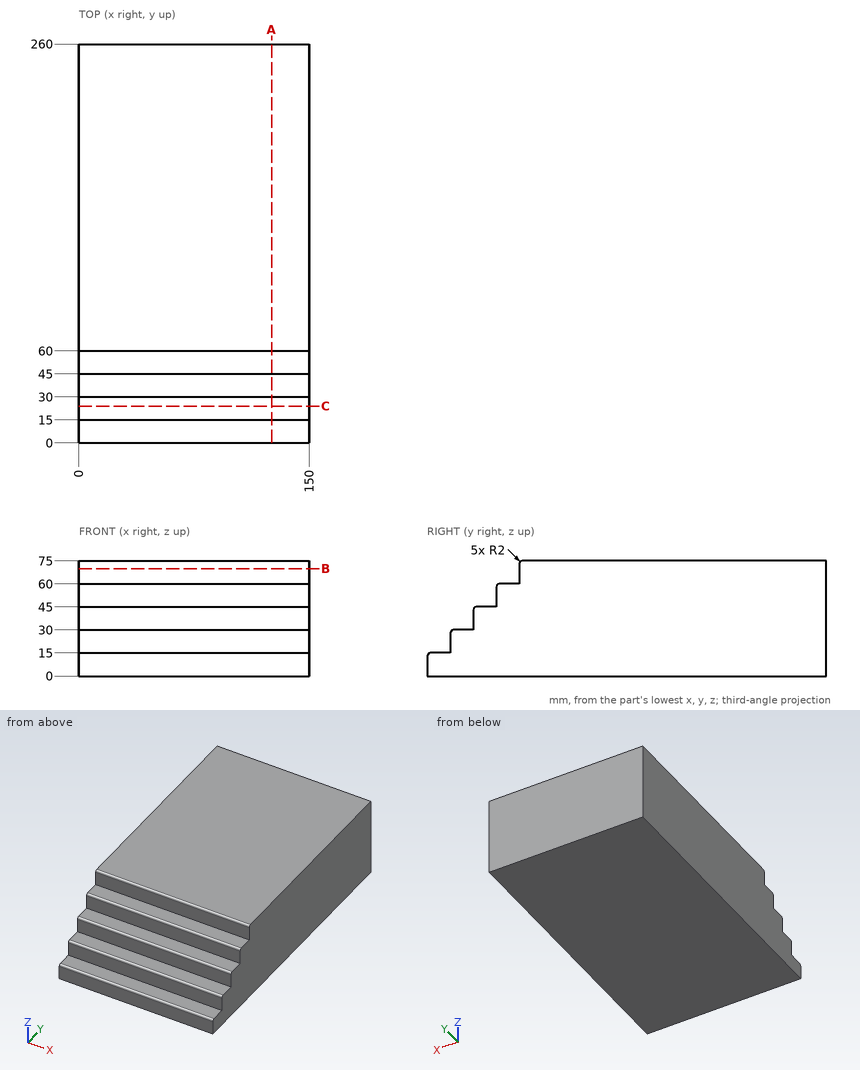
Geometry: see drawing. Coordinates: mm, zero at the bounding-box minimum. Round coordinates to 2 decimals unless told otherwise and drop trailing zeros. Write each loop counter-clockwise with the first axis right and the second up, starting at its lowest first coordinate (ties: lowest second). Pieces come first, ordered by that corner, then holes.
Item 1: Section query B-B (z = 70). Return loops of the section in (x, y), plus the area to 3 significant figures.
Item 2: Material intervals for L1, parallel to Y at x = 113.5, z = 17; L2, parallel to Y at x = 45.5, z = 71.5; L3, parallel to Z at x = 71, y = 32, sorted ascending.
Item 3: Section query A-A (x = 125.5). Return loops of the section in (y, z), plus the area to 3 significant figures.
Item 4: Section query C-C (y = 24). Return loops of the section in (x, z), plus the area to 3 significant figures.
Item 5: Pin query (flat end, axial travel): P1, Ø12, axis at x = 56.5, z = 39.5, coming from the -Y side; P2, Ø10.5, axis at x = 50.5, z = 68.5, coming from the -Y side; P3, Ø14.5, axis at x = 39, y = 11.5, coming from the +Z side. Return the tip coordinate at first contact, or that it passes through.
Completed:
1. outline: (0, 60) - (150, 60) - (150, 260) - (0, 260) - close
1. area: 30,000 mm2
2. L1: y = 15 to 260
2. L2: y = 60 to 260
2. L3: z = 0 to 45
3. outline: (0, 0) - (260, 0) - (260, 75) - (62, 75) arc R2 ccw to (60, 73) - (60, 60) - (47, 60) arc R2 ccw to (45, 58) - (45, 45) - (32, 45) arc R2 ccw to (30, 43) - (30, 30) - (17, 30) arc R2 ccw to (15, 28) - (15, 15) - (2, 15) arc R2 ccw to (0, 13) - close
3. area: 17,200 mm2
4. outline: (0, 0) - (150, 0) - (150, 30) - (0, 30) - close
4. area: 4,500 mm2
5. P1: stops at y = 30
5. P2: stops at y = 60
5. P3: stops at z = 30
